Part model, mm, in its own coordinate system. Face numbers are marked on the shaded views. A direction names the side the tool comes from. Coordinates: 2 decimals unless noted, no trailing zeros. Loops run counter-clockwise (first coordinate to the right, second up) from the corner with the lowest first, then second, coordinate; pieces in that order, holes last. Notation, with made-up numbers: (40, 7.25) -> (50, 7.25) arc R26 ccw to (50, 36.25) -> close; hole circle Ø1 at (87, 77.25). An arc over 180 degrees is marked (long way). One line per item, written item: value. Start each with the question number.
from build123d import *

# Parameters (mm, degrees)
F0_W      = 60
F0_H      = 40
F1_DEPTH  = 20
F2_W      = 60
F2_H      = 20
F3_DEPTH  = 10
F4_R      = 4
F5_DEPTH  = 25
F6_R      = 4
F7_DEPTH  = 25
F8_W      = 60
F8_H      = 5
F9_DEPTH  = 5
F10_W     = 60
F10_H     = 5
F11_DEPTH = 5
F12_R     = 1
F13_DEPTH = 5
F14_R     = 1
F15_DEPTH = 5


with BuildPart() as f1:
    # F0 (on Top) → F1 (new body)
    with BuildSketch(Plane.XY):
        Rectangle(F0_W, F0_H)
    extrude(amount=F1_DEPTH)

    # F2 (on face) → F3 (cut)
    with BuildSketch(Plane.XY.offset(20)):
        Rectangle(F2_W, F2_H)
    extrude(amount=-F3_DEPTH, mode=Mode.SUBTRACT)

    # F4 (on face) → F5 (cut)
    with BuildSketch(Plane.XY.offset(10)):
        with Locations((-16, 0)):
            Circle(F4_R)
    extrude(amount=-F5_DEPTH, mode=Mode.SUBTRACT)

    # F6 (on face) → F7 (cut)
    with BuildSketch(Plane.XY.offset(10)):
        with Locations((16, 0)):
            Circle(F6_R)
    extrude(amount=-F7_DEPTH, mode=Mode.SUBTRACT)

    # F8 (on face) → F9 (cut)
    with BuildSketch(Plane(origin=(0, 0, 0), x_dir=(1, 0, 0), z_dir=(0, 0, -1))):
        with Locations((0, 14.5)):
            Rectangle(F8_W, F8_H)
    extrude(amount=-F9_DEPTH, mode=Mode.SUBTRACT)

    # F10 (on face) → F11 (cut)
    with BuildSketch(Plane(origin=(0, 0, 0), x_dir=(1, 0, 0), z_dir=(0, 0, -1))):
        with Locations((0, -14.5)):
            Rectangle(F10_W, F10_H)
    extrude(amount=-F11_DEPTH, mode=Mode.SUBTRACT)

    # F12 (on face) → F13 (cut)
    with BuildSketch(Plane.XZ.offset(20)):
        with Locations((-26.892597, 2)):
            Circle(F12_R)
    extrude(amount=-F13_DEPTH, mode=Mode.SUBTRACT)

    # F14 (on face) → F15 (cut)
    with BuildSketch(Plane.XZ.offset(20)):
        with Locations((26, 2)):
            Circle(F14_R)
    extrude(amount=-F15_DEPTH, mode=Mode.SUBTRACT)


solid = f1.part
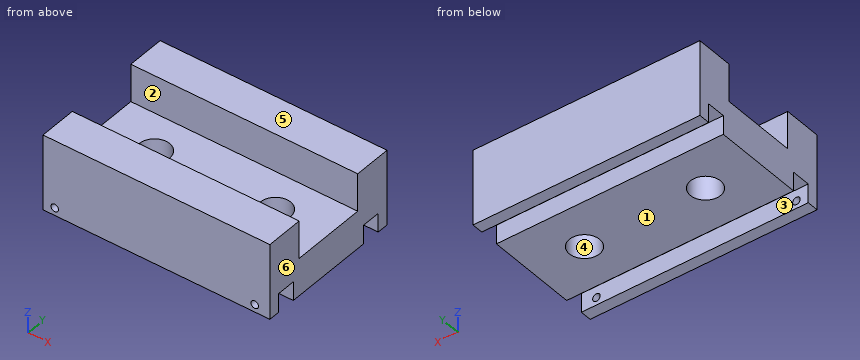
1) Slice it at D-D (x = -16). Give the cut face in (y, z), then the cut area to 3 significant figures.
2) Slice it at A-A (z = 11.25). Give the cut face in (x, y).
3) Pull direction X, two halves, no side cores. Call the marked faces 4, 5 and 6: +X half, -X half, draft (parallel to the pull), parting line (faces both ways), or undercut.
4) Probe line 1 (Y direction, x = 16, z = 2); line 2 (Y direction, x = -0.5, z = 1.75); line 3 (Z direction, x = 26, y = -19.2). List the from-to ranges inside material, lowest first. Write a range as from..to.
5) Slice it at C-C (y = 0). Give the cut face in (x, z), then the cut area to 3 significant figures.
6) Slice it at B-B (z = 2). Give the cut face in (x, y).
7) Tool access for the marked faces 1, 2 and 3: list every direction of +Z, -Z, +X, -X, +Y, -Y with a clear straight run to the whole face (end or side of a thin tool).
8) Pin check, flat tips, straight feed: pin 1 Ø7 at (x, y) = (16, 0) entering from -Z; pin 2 Ø2.5 at (x, y) = (3, -15.5) entering from -Z; pin 3 Ø1.5 at (x, y) = (0.5, -8) entering from +Z. Stop position of each tip, or through.
Check sheet entries:
1. outline: (-20, 0) -> (-17, 0) -> (-17, 5) -> (-12, 5) -> (-12, 0) -> (-4, 0) -> (-4, 10) -> (-10, 10) -> (-10, 20) -> (-20, 20) -> close; (4, 0) -> (12, 0) -> (12, 5) -> (17, 5) -> (17, 0) -> (20, 0) -> (20, 20) -> (10, 20) -> (10, 10) -> (4, 10) -> close
1. area: 470 mm^2
2. outline: (-30, -20) -> (30, -20) -> (30, -10) -> (-30, -10) -> close; (-30, 10) -> (30, 10) -> (30, 20) -> (-30, 20) -> close
3. face 4: undercut
3. face 5: draft
3. face 6: +X half
4. line 1: y = -20..-17, -12..-4, 4..12, 17..20
4. line 2: y = -20..-17, -12..12, 17..20
4. line 3: z = 0..1, 3..20
5. outline: (-30, 0) -> (-20, 0) -> (-20, 10) -> (-30, 10) -> close; (-12, 0) -> (12, 0) -> (12, 10) -> (-12, 10) -> close; (20, 0) -> (30, 0) -> (30, 10) -> (20, 10) -> close
5. area: 440 mm^2
6. outline: (-30, -20) -> (-27.89, -20) -> (-27.89, -17) -> (-30, -17) -> close; (-30, -12) -> (30, -12) -> (30, 12) -> (-30, 12) -> close; (-30, 17) -> (30, 17) -> (30, 20) -> (-30, 20) -> close; (-25.89, -20) -> (25, -20) -> (25, -17) -> (-25.89, -17) -> close; (27, -20) -> (30, -20) -> (30, -17) -> (27, -17) -> close; hole circle Ø8 at (-16, 0); hole circle Ø8 at (16, 0)
7. face 1: -Z, +X, -X, +Y, -Y
7. face 2: +Z, +X, -X
7. face 3: -Z, +X, -X
8. pin 1: passes through
8. pin 2: stops at z = 5
8. pin 3: stops at z = 10
